from build123d import *

# Parameters (mm, degrees)
SKETCH1_W           = 68
SKETCH1_H           = 50
SKETCH1_R           = 2
BOSS_EXTRUDE2_DEPTH = 2
SKETCH2_R           = 7
BOSS_EXTRUDE3_DEPTH = 28
FILLET1_R           = 0.5
SKETCH3_W           = 10
SKETCH3_H           = 38
BOSS_EXTRUDE4_DEPTH = 15
SKETCH4_W           = 15
SKETCH4_H           = 28
BOSS_EXTRUDE5_DEPTH = 10
SKETCH5_W           = 10
SKETCH5_H           = 7
BOSS_EXTRUDE6_DEPTH = 10
SKETCH6_R           = 2.75
BOSS_EXTRUDE7_DEPTH = 13
FILLET2_R           = 0.3


with BuildPart() as part:
    # Sketch1 → Boss-Extrude2 (new body)
    with BuildSketch(Plane(origin=(0, 0, 0), x_dir=(1, 0, 0), z_dir=(0, 1, 0))):
        Rectangle(SKETCH1_W, SKETCH1_H)
        with Locations(Location((-31, 22, 0), (0, 0, 270))):
            Circle(SKETCH1_R, mode=Mode.SUBTRACT)
        with Locations(Location((31, 22, 0), (0, 0, 90))):
            Circle(SKETCH1_R, mode=Mode.SUBTRACT)
        with Locations(Location((31, -22, 0), (0, 0, 270))):
            Circle(SKETCH1_R, mode=Mode.SUBTRACT)
        with Locations(Location((-31, -22, 0), (0, 0, 90))):
            Circle(SKETCH1_R, mode=Mode.SUBTRACT)
    extrude(amount=BOSS_EXTRUDE2_DEPTH)

    # Sketch2 → Boss-Extrude3 (add)
    with BuildSketch(Plane(origin=(0, 2, 0), x_dir=(1, 0, 0), z_dir=(0, 1, 0))):
        with Locations(Location((16, 0, 0), (0, 0, 90))):
            Circle(SKETCH2_R)
    extrude(amount=BOSS_EXTRUDE3_DEPTH)

    # Fillet1
    fillet1_edges = [part.edges().sort_by_distance(p)[0] for p in [
        (16, 30, 7),
    ]]
    fillet(fillet1_edges, radius=FILLET1_R)

    # Sketch3 → Boss-Extrude4 (add)
    with BuildSketch(Plane(origin=(0, 2, 0), x_dir=(1, 0, 0), z_dir=(0, 1, 0))):
        with Locations((29, 0)):
            Rectangle(SKETCH3_W, SKETCH3_H)
    extrude(amount=BOSS_EXTRUDE4_DEPTH)

    # Sketch4 → Boss-Extrude5 (add)
    with BuildSketch(Plane(origin=(0, 2, 0), x_dir=(1, 0, 0), z_dir=(0, 1, 0))):
        with Locations((-26.5, 0)):
            Rectangle(SKETCH4_W, SKETCH4_H)
    extrude(amount=BOSS_EXTRUDE5_DEPTH)

    # Sketch5 → Boss-Extrude6 (add)
    with BuildSketch(Plane(origin=(0, 2, 0), x_dir=(1, 0, 0), z_dir=(0, 1, 0))):
        with Locations((-23.001541076, 21.262939999)):
            Rectangle(SKETCH5_W, SKETCH5_H)
    extrude(amount=BOSS_EXTRUDE6_DEPTH)

    # Sketch6 → Boss-Extrude7 (add)
    with BuildSketch(Plane(origin=(0, 2, 0), x_dir=(1, 0, 0), z_dir=(0, 1, 0))):
        with Locations(Location((-14, 21.411376653, 0), (0, 0, 90))):
            Circle(SKETCH6_R)
    extrude(amount=BOSS_EXTRUDE7_DEPTH)

    # Fillet2
    fillet2_edges = [part.edges().sort_by_distance(p)[0] for p in [
        (-14, 15, -18.661376653),
    ]]
    fillet(fillet2_edges, radius=FILLET2_R)


solid = part.part
The model under review builds one solid part; all positions refer to its coordinate system, in mm. A direction names the side the tool comes from. Round coordinates to 2 decimals unless told otherwise and drop trailing zeros. Loops run counter-clockwise (first coordinate to the right, second up) from the corner with the lowest first, then second, coordinate; pieces in that order, holes last. Notation, with made-up numbers: (59.25, -11.75) -> (109.25, -11.75) arc R9 ccw to (109.25, -7.75) -> close; hole circle Ø1 at (44, 27.25). An arc over 180 degrees is marked (long way). Write item = value, one per line. Start each with the question number.
Item 1: Mouldability with a two-part tool opening along X and no side actions: class faces 1 (the cylindrical face through (-29, 1, 22)), 2 (the flat face through (34, 8, 0)), 3 (the flat face through (-27, 12, 0)), 4 (the cylindrical face through (-33, 1, -22)) as released by +X, released by -X, zero draft, split by the parting line, or undercut.
Item 2: Take a section at A-A on x = 31. Give the boundary of the cut face in (y, z).
Item 3: Take a section at D-D on x = -31. Give the boundary of the cut face in (y, z).
Item 4: To check wall thickness, follow L1, parallel to X at y = 1.65, z = 22; L2, parallel to Z at x = -21.5, y = 9.75; L3, parallel to Y at x = -27.5, z = 13. State the ranges of each line that lie inside material, in increasing order.
Item 5: Insertion check: pin 1 (1 mm diameter, centred on y = 26, z = -1, fed in from -X); pin 2 (2 mm diameter, centred on y = 5, z = -22, fed in from -X); pin 3 (5 mm diameter, centred on x = 29.5, y = 8, fed in from -Z); pin 4 (3 mm diameter, centred on x = 31, z = 22, fed in from +Y). Each pin has a flat end and moves straight along its axis. Give the tip position at first contact, or say it passes through.
Item 6: For faces 5 (the flat face through (-27, 7, -14)), 6 (the flat face through (29, 9, 19)), 7 (the flat face through (-19, 7, 0)), list the 3-axis set-ups (+Z, -Z, +X, -X, +Y, -Y) from which the entire face can be reached by the end or side of a thin tool; tool diameter is ignored.
Item 7: Take a section at C-C on z = 8.5. Give the boundary of the cut face in (x, y).
Item 8: Take a section at B-B on y = 9.25. Give the boundary of the cut face in (x, z).
Result:
q1.face_1 = undercut
q1.face_2 = released by +X
q1.face_3 = zero draft
q1.face_4 = undercut
q2.outline = (0, -25) -> (2, -25) -> (2, -24) -> (0, -24) -> close; (0, -20) -> (2, -20) -> (2, -19) -> (17, -19) -> (17, 19) -> (2, 19) -> (2, 20) -> (0, 20) -> close; (0, 24) -> (2, 24) -> (2, 25) -> (0, 25) -> close
q3.outline = (0, -25) -> (2, -25) -> (2, -24) -> (0, -24) -> close; (0, -20) -> (2, -20) -> (2, -14) -> (12, -14) -> (12, 14) -> (2, 14) -> (2, 20) -> (0, 20) -> close; (0, 24) -> (2, 24) -> (2, 25) -> (0, 25) -> close
q4.L1 = -34 to -33, -29 to 29, 33 to 34
q4.L2 = -24.76 to -17.76, -14 to 14
q4.L3 = 0 to 12
q5.pin_1 = 9.02
q5.pin_2 = -28
q5.pin_3 = -19
q5.pin_4 = through
q6.face_5 = -X, +Y
q6.face_6 = +Z, +X, -X, +Y
q6.face_7 = +Z, +Y
q7.outline = (-34, 0) -> (34, 0) -> (34, 17) -> (24, 17) -> (24, 2) -> (-19, 2) -> (-19, 12) -> (-34, 12) -> close
q8.outline = (-34, -14) -> (-19, -14) -> (-19, 14) -> (-34, 14) -> close; (-28, -24.76) -> (-18, -24.76) -> (-18, -17.76) -> (-28, -17.76) -> close; circle Ø5.5 at (-14, -21.41); circle Ø14 at (16, 0); (24, -19) -> (34, -19) -> (34, 19) -> (24, 19) -> close
